```python
from build123d import *

# Parameters (mm, degrees)
SKETCH1_W                               = 51
SKETCH1_H                               = 31
BOSS_EXTRUDE1_DEPTH                     = 8
SKETCH5_W                               = 31
SKETCH5_H                               = 14
BOSS_EXTRUDE3_DEPTH                     = 30
CUT_EXTRUDE3_DEPTH                      = 68.977937597
FILLET1_R                               = 10
SKETCH8_R                               = 1.75
F_3_5MM_SCREW_HOLE_FOR_TENSIONING_DEPTH = 64.921827371


with BuildPart() as part:
    # Sketch1 → Boss-Extrude1 (new body)
    with BuildSketch(Plane(origin=(0, 0, 0), x_dir=(1, 0, 0), z_dir=(0, 1, 0))):
        with Locations((25.5, 15.5)):
            Rectangle(SKETCH1_W, SKETCH1_H)
    extrude(amount=BOSS_EXTRUDE1_DEPTH)

    # Sketch5 → Boss-Extrude3 (add)
    with BuildSketch(Plane(origin=(0, 8, 0), x_dir=(1, 0, 0), z_dir=(0, 1, 0))):
        with Locations((25.5, 17)):
            Rectangle(SKETCH5_W, SKETCH5_H)
    extrude(amount=BOSS_EXTRUDE3_DEPTH)

    # Sketch6 → Cut-Extrude3 (cut, through all)
    with BuildSketch(Plane(origin=(0, 0, -24), x_dir=(-1, 0, 0), z_dir=(0, 0, -1))):
        with BuildLine():
            Line((-32.000000097, 30.65), (-18.999999903, 30.65))
            ThreePointArc((-18.999999903, 30.65), (-16.499999903, 28.15), (-18.999999903, 25.65))
            Line((-18.999999903, 25.65), (-32.000000097, 25.65))
            ThreePointArc((-32.000000097, 25.65), (-34.500000097, 28.15), (-32.000000097, 30.65))
        make_face()
    extrude(amount=-CUT_EXTRUDE3_DEPTH, mode=Mode.SUBTRACT)

    # Fillet1
    # the kernel refuses this fillet: 10 mm, written as the material it adds along each edge
    with BuildSketch(Plane(origin=(41, 8, -24), x_dir=(0, 0, -1), z_dir=(-1, 0, 0))) as fillet1_piece_1:
        with BuildLine():
            CenterArc((10, -9.539392014), FILLET1_R, 107.457603124, 72.542396876)
            Line((0, -9.539392014), (-0.2, -9.539392014))
            Line((-0.2, -9.539392014), (-0.2, 0))
            Line((-0.2, 0), (0, 0.2))
            ThreePointArc((0, 0.2), (3.5, 0.2), (6.94, 0.19078784))
            Line((6.94, 0.19078784), (7, 0))
        make_face()
    extrude(amount=31)
    with BuildSketch(Plane(origin=(10, 8, -24), x_dir=(-1, 0, 0), z_dir=(0, 0, 1)), Plane(origin=(41, 8, -10), x_dir=(1, 0, 0), z_dir=(0, 0, -1))) as fillet1_piece_2:
        with BuildLine():
            CenterArc((FILLET1_R, -FILLET1_R), FILLET1_R, 90, 90)
            Line((0, -FILLET1_R), (-FILLET1_R * 0.02, -FILLET1_R))
            Line((-FILLET1_R * 0.02, -FILLET1_R), (-FILLET1_R * 0.02, FILLET1_R * 0.02))
            Line((-FILLET1_R * 0.02, FILLET1_R * 0.02), (FILLET1_R, FILLET1_R * 0.02))
            Line((FILLET1_R, FILLET1_R * 0.02), (FILLET1_R, 0))
        make_face()
    extrude(amount=14)
    with BuildSketch(Plane(origin=(10, 8, -10), x_dir=(0, 0, 1), z_dir=(1, 0, 0))) as fillet1_piece_3:
        with BuildLine():
            CenterArc((FILLET1_R, -FILLET1_R), FILLET1_R, 90, 90)
            Line((0, -FILLET1_R), (-FILLET1_R * 0.02, -FILLET1_R))
            Line((-FILLET1_R * 0.02, -FILLET1_R), (-FILLET1_R * 0.02, FILLET1_R * 0.02))
            Line((-FILLET1_R * 0.02, FILLET1_R * 0.02), (FILLET1_R, FILLET1_R * 0.02))
            Line((FILLET1_R, FILLET1_R * 0.02), (FILLET1_R, 0))
        make_face()
    extrude(amount=31)
    with BuildSketch(Plane(origin=(64.848480035, 8, -24), x_dir=(0, 0, -1), z_dir=(-1, 0, 0))) as fillet1_piece_4a_section:
        with BuildLine():
            CenterArc((10, -9.539392014), FILLET1_R, 107.457603124, 72.542396876)
            Line((0, -9.539392014), (-0.2, -9.539392014))
            Line((-0.2, -9.539392014), (-0.2, 0))
            Line((-0.2, 0), (0, 0.2))
            ThreePointArc((0, 0.2), (3.5, 0.2), (6.94, 0.19078784))
            Line((6.94, 0.19078784), (7, 0))
        make_face()
    fillet1_piece_4a = extrude(amount=54.848480035, mode=Mode.PRIVATE)
    fillet1_piece_4a = split(fillet1_piece_4a, bisect_by=Plane(origin=(51, 10.271225878, -25.787817996), z_dir=(-1, 0, 0)), keep=Keep.TOP, mode=Mode.PRIVATE)
    fillet1_piece_4a = split(fillet1_piece_4a, bisect_by=Plane(origin=(41, 10.271225878, -25.787817996), z_dir=(1, 0, 0)), keep=Keep.TOP, mode=Mode.PRIVATE)
    with BuildSketch(Plane(origin=(41, 8, -10), x_dir=(1, 0, 0), z_dir=(0, 0, -1))) as fillet1_piece_4b_section:
        with BuildLine():
            CenterArc((FILLET1_R, -FILLET1_R), FILLET1_R, 90, 90)
            Line((0, -FILLET1_R), (-FILLET1_R * 0.02, -FILLET1_R))
            Line((-FILLET1_R * 0.02, -FILLET1_R), (-FILLET1_R * 0.02, FILLET1_R * 0.02))
            Line((-FILLET1_R * 0.02, FILLET1_R * 0.02), (FILLET1_R, FILLET1_R * 0.02))
            Line((FILLET1_R, FILLET1_R * 0.02), (FILLET1_R, 0))
        make_face()
    fillet1_piece_4b = extrude(amount=39, mode=Mode.PRIVATE)
    fillet1_piece_4b = split(fillet1_piece_4b, bisect_by=Plane(origin=(43.263951143, 10.263951143, -31), z_dir=(0, 0, 1)), keep=Keep.TOP, mode=Mode.PRIVATE)
    fillet1_piece_4b = split(fillet1_piece_4b, bisect_by=Plane(origin=(43.263951143, 10.263951143, -24), z_dir=(0, 0, -1)), keep=Keep.TOP, mode=Mode.PRIVATE)
    fillet1_piece_4 = fillet1_piece_4a & fillet1_piece_4b
    add(fillet1_piece_4)
    with BuildSketch(Plane(origin=(41, 8, -24), x_dir=(0, 0, -1), z_dir=(-1, 0, 0))) as fillet1_piece_5a_section:
        with BuildLine():
            CenterArc((10, -9.539392014), FILLET1_R, 107.457603124, 72.542396876)
            Line((0, -9.539392014), (-0.2, -9.539392014))
            Line((-0.2, -9.539392014), (-0.2, 0))
            Line((-0.2, 0), (0, 0.2))
            ThreePointArc((0, 0.2), (3.5, 0.2), (6.94, 0.19078784))
            Line((6.94, 0.19078784), (7, 0))
        make_face()
    fillet1_piece_5a = extrude(amount=54.848480035, mode=Mode.PRIVATE)
    fillet1_piece_5a = split(fillet1_piece_5a, bisect_by=Plane(origin=(0, 10.271225878, -25.787817996), z_dir=(1, 0, 0)), keep=Keep.TOP, mode=Mode.PRIVATE)
    fillet1_piece_5a = split(fillet1_piece_5a, bisect_by=Plane(origin=(10, 10.271225878, -25.787817996), z_dir=(-1, 0, 0)), keep=Keep.TOP, mode=Mode.PRIVATE)
    with BuildSketch(Plane(origin=(10, 8, -49), x_dir=(-1, 0, 0), z_dir=(0, 0, 1))) as fillet1_piece_5b_section:
        with BuildLine():
            CenterArc((FILLET1_R, -FILLET1_R), FILLET1_R, 90, 90)
            Line((0, -FILLET1_R), (-FILLET1_R * 0.02, -FILLET1_R))
            Line((-FILLET1_R * 0.02, -FILLET1_R), (-FILLET1_R * 0.02, FILLET1_R * 0.02))
            Line((-FILLET1_R * 0.02, FILLET1_R * 0.02), (FILLET1_R, FILLET1_R * 0.02))
            Line((FILLET1_R, FILLET1_R * 0.02), (FILLET1_R, 0))
        make_face()
    fillet1_piece_5b = extrude(amount=39, mode=Mode.PRIVATE)
    fillet1_piece_5b = split(fillet1_piece_5b, bisect_by=Plane(origin=(7.736048857, 10.263951143, -31), z_dir=(0, 0, 1)), keep=Keep.TOP, mode=Mode.PRIVATE)
    fillet1_piece_5b = split(fillet1_piece_5b, bisect_by=Plane(origin=(7.736048857, 10.263951143, -24), z_dir=(0, 0, -1)), keep=Keep.TOP, mode=Mode.PRIVATE)
    fillet1_piece_5 = fillet1_piece_5a & fillet1_piece_5b
    add(fillet1_piece_5)
    with BuildSketch(Plane(origin=(10, 8, -24), x_dir=(-1, 0, 0), z_dir=(0, 0, 1))) as fillet1_piece_6a_section:
        with BuildLine():
            CenterArc((FILLET1_R, -FILLET1_R), FILLET1_R, 90, 90)
            Line((0, -FILLET1_R), (-FILLET1_R * 0.02, -FILLET1_R))
            Line((-FILLET1_R * 0.02, -FILLET1_R), (-FILLET1_R * 0.02, FILLET1_R * 0.02))
            Line((-FILLET1_R * 0.02, FILLET1_R * 0.02), (FILLET1_R, FILLET1_R * 0.02))
            Line((FILLET1_R, FILLET1_R * 0.02), (FILLET1_R, 0))
        make_face()
    fillet1_piece_6a = extrude(amount=39, mode=Mode.PRIVATE)
    fillet1_piece_6a = split(fillet1_piece_6a, bisect_by=Plane(origin=(7.736048857, 10.263951143, 0), z_dir=(0, 0, -1)), keep=Keep.TOP, mode=Mode.PRIVATE)
    fillet1_piece_6a = split(fillet1_piece_6a, bisect_by=Plane(origin=(7.736048857, 10.263951143, -10), z_dir=(0, 0, 1)), keep=Keep.TOP, mode=Mode.PRIVATE)
    with BuildSketch(Plane(origin=(-15, 8, -10), x_dir=(0, 0, 1), z_dir=(1, 0, 0))) as fillet1_piece_6b_section:
        with BuildLine():
            CenterArc((FILLET1_R, -FILLET1_R), FILLET1_R, 90, 90)
            Line((0, -FILLET1_R), (-FILLET1_R * 0.02, -FILLET1_R))
            Line((-FILLET1_R * 0.02, -FILLET1_R), (-FILLET1_R * 0.02, FILLET1_R * 0.02))
            Line((-FILLET1_R * 0.02, FILLET1_R * 0.02), (FILLET1_R, FILLET1_R * 0.02))
            Line((FILLET1_R, FILLET1_R * 0.02), (FILLET1_R, 0))
        make_face()
    fillet1_piece_6b = extrude(amount=56, mode=Mode.PRIVATE)
    fillet1_piece_6b = split(fillet1_piece_6b, bisect_by=Plane(origin=(0, 10.263951143, -7.736048857), z_dir=(1, 0, 0)), keep=Keep.TOP, mode=Mode.PRIVATE)
    fillet1_piece_6b = split(fillet1_piece_6b, bisect_by=Plane(origin=(10, 10.263951143, -7.736048857), z_dir=(-1, 0, 0)), keep=Keep.TOP, mode=Mode.PRIVATE)
    fillet1_piece_6 = fillet1_piece_6a & fillet1_piece_6b
    add(fillet1_piece_6)
    with BuildSketch(Plane(origin=(10, 8, -10), x_dir=(0, 0, 1), z_dir=(1, 0, 0))) as fillet1_piece_7a_section:
        with BuildLine():
            CenterArc((FILLET1_R, -FILLET1_R), FILLET1_R, 90, 90)
            Line((0, -FILLET1_R), (-FILLET1_R * 0.02, -FILLET1_R))
            Line((-FILLET1_R * 0.02, -FILLET1_R), (-FILLET1_R * 0.02, FILLET1_R * 0.02))
            Line((-FILLET1_R * 0.02, FILLET1_R * 0.02), (FILLET1_R, FILLET1_R * 0.02))
            Line((FILLET1_R, FILLET1_R * 0.02), (FILLET1_R, 0))
        make_face()
    fillet1_piece_7a = extrude(amount=56, mode=Mode.PRIVATE)
    fillet1_piece_7a = split(fillet1_piece_7a, bisect_by=Plane(origin=(51, 10.263951143, -7.736048857), z_dir=(-1, 0, 0)), keep=Keep.TOP, mode=Mode.PRIVATE)
    fillet1_piece_7a = split(fillet1_piece_7a, bisect_by=Plane(origin=(41, 10.263951143, -7.736048857), z_dir=(1, 0, 0)), keep=Keep.TOP, mode=Mode.PRIVATE)
    with BuildSketch(Plane(origin=(41, 8, 15), x_dir=(1, 0, 0), z_dir=(0, 0, -1))) as fillet1_piece_7b_section:
        with BuildLine():
            CenterArc((FILLET1_R, -FILLET1_R), FILLET1_R, 90, 90)
            Line((0, -FILLET1_R), (-FILLET1_R * 0.02, -FILLET1_R))
            Line((-FILLET1_R * 0.02, -FILLET1_R), (-FILLET1_R * 0.02, FILLET1_R * 0.02))
            Line((-FILLET1_R * 0.02, FILLET1_R * 0.02), (FILLET1_R, FILLET1_R * 0.02))
            Line((FILLET1_R, FILLET1_R * 0.02), (FILLET1_R, 0))
        make_face()
    fillet1_piece_7b = extrude(amount=39, mode=Mode.PRIVATE)
    fillet1_piece_7b = split(fillet1_piece_7b, bisect_by=Plane(origin=(43.263951143, 10.263951143, 0), z_dir=(0, 0, -1)), keep=Keep.TOP, mode=Mode.PRIVATE)
    fillet1_piece_7b = split(fillet1_piece_7b, bisect_by=Plane(origin=(43.263951143, 10.263951143, -10), z_dir=(0, 0, 1)), keep=Keep.TOP, mode=Mode.PRIVATE)
    fillet1_piece_7 = fillet1_piece_7a & fillet1_piece_7b
    add(fillet1_piece_7)

    # Sketch8 → 3.5mm screw hole for tensioning (cut, through all)
    with BuildSketch(Plane(origin=(41, 0, 0), x_dir=(0, 0, -1), z_dir=(1, 0, 0))):
        with Locations((17, 28.15)):
            Circle(SKETCH8_R)
    extrude(amount=-F_3_5MM_SCREW_HOLE_FOR_TENSIONING_DEPTH, mode=Mode.SUBTRACT)


solid = part.part
```
Work out the finished part from the listing and answer in its coordinate system (mm). A direction names the side the tool comes from. Give positions to 0.01 mm unless a question says otherwise; leave off trailing zeros. Order: outer loops, then holes, each group sorted by start corner. A loop starts at its lowest first (then second) coordinate and runs counter-clockwise, first axis right, second up. Notation, with made-up numbers: (35, 37.25) - (52, 37.25) arc R34 ccw to (52, 68.25) - close; hole circle Ø10 at (-11, 21). An arc over 180 degrees is marked (long way). One line per item, written item: value. Start each with the question number.
1. Each of these flat-tipped pins is pushed along its axis until it touches: pin 1 Ø4 at (y, z) = (26.5, -19.5) entering from -X; pin 2 Ø3 at (y, z) = (28.15, -17) entering from +X; pin 3 Ø1 at (x, y) = (17.5, 31.5) entering from -Z; pin 4 Ø22 at (x, y) = (18, 28.5) entering from +Z. Where does it stop, or does it pass through?
2. Section D-D, the plane y = 23.5 is taken. Write down the section's boundary in (x, z).
3. Which of the six approach directions +Z, -Z, +X, -X, +Y, -Y give full straight-line access (tool end or side, diameter ignored) to faces 1 (the face through (41, 30.1, -17.1)), 2 (the face through (25, 25, -24)), 3 (the face through (26, 30.65, -17)), 4 (the face through (10, 30.1, -17.1))?
4. For a pull along Y with two mould halves and no side action, classify faces 5 (the face through (25, 4, 0)), 6 (the face through (6, 10, -16)), 7 (the face through (17.703, 26.013, -17.098)), 8 (the face through (25, 25.65, -17)) as released by +Y, released by -Y, zero draft, split by the parting line, or undercut.
5. Section B-B, the plane x = 35.5 is taken. Write down the section's boundary in (y, z), then the cut area to 3 significant figures.
6. Consider line 1 (Y direction, x = 13, z = -17); line 2 (Z direction, x = 36.5, y = 28.15); line 3 (Y direction, x = 21, z = -15). Determine where each line is inside the solid, lowest interval first.
7. Section C-C, the plane z = -18 is taken. Write down the section's boundary in (x, y), then the cut area to 3 significant figures.
8. Section A-A, the plane y = 28.15 is taken. Write down the section's boundary in (x, z).
Filled sheet:
1. pin 1: x = 10
1. pin 2: through
1. pin 3: z = -24
1. pin 4: z = -9.99
2. outline: (10, -24) - (41, -24) - (41, -10) - (10, -10) - close
3. face 1: +Z, -Z, +X, +Y
3. face 2: -Z, +X, -X, +Y
3. face 3: +Z, -Z
3. face 4: +Z, -Z, -X, +Y
4. face 5: zero draft
4. face 6: released by +Y
4. face 7: undercut
4. face 8: undercut
5. outline: (0, -31) - (8, -31) arc R10 cw to (17.54, -24) - (38, -24) - (38, -10) - (18, -10) arc R10 cw to (8, 0) - (0, 0) - close; hole circle Ø3.5 at (28.15, -17)
5. area: 698 mm²
6. line 1: 0 to 26.4, 29.9 to 38
6. line 2: -24 to -18.75, -15.25 to -10
6. line 3: 0 to 25.65, 30.65 to 38
7. outline: (0, 0) - (51, 0) - (51, 8) arc R10 cw to (41, 18) - (41, 26.71) - (34.05, 26.71) arc R2.5 cw to (32, 25.65) - (19, 25.65) arc R2.5 cw to (16.95, 26.71) - (10, 26.71) - (10, 18) arc R10 cw to (0, 8) - close; (10, 29.59) - (16.95, 29.59) arc R2.5 cw to (19, 30.65) - (32, 30.65) arc R2.5 cw to (34.05, 29.59) - (41, 29.59) - (41, 38) - (10, 38) - close
7. area: 1,260 mm²
8. outline: (10, -24) - (16.5, -24) - (16.5, -18.75) - (10, -18.75) - close; (10, -15.25) - (16.5, -15.25) - (16.5, -10) - (10, -10) - close; (34.5, -24) - (41, -24) - (41, -18.75) - (34.5, -18.75) - close; (34.5, -15.25) - (41, -15.25) - (41, -10) - (34.5, -10) - close
